The listing builds one solid part. Answer for the finished solid, in the listing's coordinates (mm). Coordinates: 2 decimals unless noted, no trailing zeros. Order: outer loops, then holes, each group sorted by start corner. A loop starts at its lowest first (then second) coordinate and runs counter-clockwise, first axis right, second up. Notation, with made-up numbers: (51.25, 28) -> (62.25, 28) arc R9 cw to (62.25, 42) -> close; hole circle Ø1 at (21.5, 30.5). An arc over 180 degrees is marked (long way). Answer in a Markdown table with one row per item.
```python
from build123d import *

# Parameters (mm, degrees)
SKETCH1_W           = 313
SKETCH1_H           = 342
BOSS_EXTRUDE1_DEPTH = 6.35
SKETCH3_W           = 22
SKETCH3_H           = 155.14040353
SKETCH3_R           = 2.5
BOSS_EXTRUDE2_DEPTH = 6.35
SKETCH2_R           = 2.5
CUT_EXTRUDE1_DEPTH  = 7.35
SKETCH4_R           = 3.5
CUT_EXTRUDE2_DEPTH  = 7.35
CUT_EXTRUDE3_DEPTH  = 7.35


with BuildPart() as part:
    # Sketch1 → Boss-Extrude1 (new body)
    with BuildSketch(Plane(origin=(0, 0, 0), x_dir=(1, 0, 0), z_dir=(0, 1, 0))):
        Rectangle(SKETCH1_W, SKETCH1_H)
    extrude(amount=-BOSS_EXTRUDE1_DEPTH)

    # Sketch3 → Boss-Extrude2 (add)
    with BuildSketch(Plane(origin=(0, 0, 0), x_dir=(1, 0, 0), z_dir=(0, 1, 0))):
        with Locations((167.5, 9)):
            Rectangle(SKETCH3_W, SKETCH3_H)
        with Locations((166.5, 9)):
            Circle(SKETCH3_R, mode=Mode.SUBTRACT)
        with Locations((166.5, -41.8)):
            Circle(SKETCH3_R, mode=Mode.SUBTRACT)
        with Locations((166.5, 59.8)):
            Circle(SKETCH3_R, mode=Mode.SUBTRACT)
    extrude(amount=-BOSS_EXTRUDE2_DEPTH)

    # Sketch2 → Cut-Extrude1 (cut, through all)
    with BuildSketch(Plane(origin=(0, 0, 0), x_dir=(1, 0, 0), z_dir=(0, 1, 0))):
        with Locations((0, -123)):
            Circle(SKETCH2_R)
        with Locations((-70, -123)):
            Circle(SKETCH2_R)
        with Locations((70, -123)):
            Circle(SKETCH2_R)
        with Locations((-70, 141)):
            Circle(SKETCH2_R)
        with Locations((0, 141)):
            Circle(SKETCH2_R)
        with Locations((70, 141)):
            Circle(SKETCH2_R)
    extrude(amount=-CUT_EXTRUDE1_DEPTH, mode=Mode.SUBTRACT)

    # Sketch4 → Cut-Extrude2 (cut, through all)
    with BuildSketch(Plane(origin=(0, 0, 0), x_dir=(1, 0, 0), z_dir=(0, 1, 0))):
        with Locations((133.64, 160.84)):
            Circle(SKETCH4_R)
        with Locations((108.24, 160.84)):
            Circle(SKETCH4_R)
    cut_extrude2 = extrude(amount=-CUT_EXTRUDE2_DEPTH, mode=Mode.SUBTRACT)

    # Mirror1: Cut-Extrude2 across plane
    add(cut_extrude2.mirror(Plane(origin=(0, 0, -9), x_dir=(1, 0, 0), z_dir=(0, 0, -1))), mode=Mode.SUBTRACT)

    # Sketch5 → Cut-Extrude3 (cut, through all)
    with BuildSketch(Plane(origin=(0, 0, 0), x_dir=(1, 0, 0), z_dir=(0, 1, 0))):
        Polygon((139.671773243, 36.673783491), (147.171773243, 36.673783491), (147.143523721, -23.326216509), (139.643523721, -23.326216509), align=None)
    extrude(amount=-CUT_EXTRUDE3_DEPTH, mode=Mode.SUBTRACT)


solid = part.part
```
(1) Find the intervals of material crossed by line 1 along X through (y, z) = (-2.25, 123); line 2 along Z through (x, y) = (0, -1.25); line 3 along X through (y, z) = (-2.25, 142.84), in increasing order. Write a range as from..to.
Check values:
| item | result |
|---|---|
| line 1 | -156.5..-72.5, -67.5..-2.5, 2.5..67.5, 72.5..156.5 |
| line 2 | -171..-143.5, -138.5..120.5, 125.5..171 |
| line 3 | -156.5..104.74, 111.74..130.14, 137.14..156.5 |
(2) A cutting plane is placed at A-A, the plane y = -3.5. Count the separate pieces of the cut face and the enclosed holes in it, then the cut area to 3 significant figures.
Check values:
| item | result |
|---|---|
| separate pieces | 1 |
| enclosed holes | 14 |
| area | 110,000 mm² |
(3) A cutting plane is placed at B-B, the plane z = -131.5. Determine the outline of the cut face in (x, y), then the cut area to 3 significant figures.
Check values:
| item | result |
|---|---|
| outline | (-156.5, -6.35) -> (156.5, -6.35) -> (156.5, 0) -> (-156.5, 0) -> close |
| area | 1,990 mm² |
(4) Flat-ended cylindrical pins translate along their axes: pin 1 (3 mm diameter, centred on y = -4.5, z = 134, fed in from +X); pin 2 (4.5 mm diameter, centred on x = -70, z = -141, fed in from -Y); pin 3 (3 mm diameter, centred on x = 170, y = -2.5, fed in from +Z); pin 4 (5 mm diameter, centred on x = -18.5, z = 26.5, fed in from +Y). Find the tip coordinate at first contact, or state that the pin passes through.
Check values:
| item | result |
|---|---|
| pin 1 | x = 156.5 |
| pin 2 | through |
| pin 3 | z = 68.57 |
| pin 4 | y = 0 |
